from build123d import *

# Parameters (mm, degrees)
CYLINDER948_R           = 0.9
CYLINDER948_DEPTH       = 15
CYLINDER948_ROLL_ANGLE  = 90
CYLINDER949_R           = 0.9
CYLINDER949_DEPTH       = 15
CYLINDER949_ROLL_ANGLE  = 90
CYLINDER947_R           = 1.25
CYLINDER947_DEPTH       = 10
CYLINDER947_PITCH_ANGLE = 90
CYLINDER946_R           = 1.25
CYLINDER946_DEPTH       = 10
CYLINDER946_PITCH_ANGLE = 90
BOX556_W                = 8
BOX556_H                = 15
BOX556_DEPTH            = 20


with BuildPart() as cylinder1099:
    # Cylinder948 → Cylinder948 (new body)
    with BuildSketch(Plane.XY):
        Circle(CYLINDER948_R)
    extrude(amount=CYLINDER948_DEPTH)


with BuildPart() as cylinder1099_1:
    # Cylinder948 roll: moved
    add(cylinder1099.part.rotate(Axis((0, 0, 0), (1, 0, 0)), CYLINDER948_ROLL_ANGLE))


with BuildPart() as cylinder1099_2:
    # Cylinder948 placement: moved
    add(cylinder1099_1.part.moved(Location((27, 85, -10.2))))


with BuildPart() as fusion595:
    # Cylinder949 → Cylinder949 (new body)
    with BuildSketch(Plane.XY):
        Circle(CYLINDER949_R)
    extrude(amount=CYLINDER949_DEPTH)


with BuildPart() as fusion595_1:
    # Cylinder949 roll: moved
    add(fusion595.part.rotate(Axis((0, 0, 0), (1, 0, 0)), CYLINDER949_ROLL_ANGLE))


with BuildPart() as fusion595_2:
    # Cylinder949 placement: moved
    add(fusion595_1.part.moved(Location((27, 85, 0))))

    # Fusion595: union Cylinder1099
    add(cylinder1099_2.part)


with BuildPart() as fusion595_3:
    # Fusion595 placement: moved
    add(fusion595_2.part.moved(Location((-4.2, 9.5, -5.9))))


with BuildPart() as cylinder1094:
    # Cylinder947 → Cylinder947 (new body)
    with BuildSketch(Plane.XY):
        Circle(CYLINDER947_R)
    extrude(amount=CYLINDER947_DEPTH)


with BuildPart() as cylinder1094_1:
    # Cylinder947 pitch: moved
    add(cylinder1094.part.rotate(Axis((0, 0, 0), (0, 1, 0)), CYLINDER947_PITCH_ANGLE))


with BuildPart() as cylinder1094_2:
    # Cylinder947 placement: moved
    add(cylinder1094_1.part.moved(Location((13.5, 83, -11))))


with BuildPart() as fusion594:
    # Cylinder946 → Cylinder946 (new body)
    with BuildSketch(Plane.XY):
        Circle(CYLINDER946_R)
    extrude(amount=CYLINDER946_DEPTH)


with BuildPart() as fusion594_1:
    # Cylinder946 pitch: moved
    add(fusion594.part.rotate(Axis((0, 0, 0), (0, 1, 0)), CYLINDER946_PITCH_ANGLE))


with BuildPart() as fusion594_2:
    # Cylinder946 placement: moved
    add(fusion594_1.part.moved(Location((13.5, 91, -11))))

    # Fusion594: union Cylinder1094
    add(cylinder1094_2.part)


with BuildPart() as fusion594_3:
    # Fusion594 placement: moved
    add(fusion594_2.part.moved(Location((4, 0, 0))))


with BuildPart() as steering_servo_front_mount:
    # Box556 → Box556 (new body)
    with BuildSketch(Plane(origin=(19.5, 79.5, -21), x_dir=(1, 0, 0), z_dir=(0, 0, 1))):
        with Locations((4, 7.5)):
            Rectangle(BOX556_W, BOX556_H)
    extrude(amount=BOX556_DEPTH)

    # Cut693: cut Fusion594
    add(fusion594_3.part, mode=Mode.SUBTRACT)

    # Cut694: cut Fusion595
    add(fusion595_3.part, mode=Mode.SUBTRACT)


solid = steering_servo_front_mount.part
For this review, take the finished solid that the model builds, in its own axes (mm). Coordinates: 2 decimals unless noted, no trailing zeros. Order: outer loops, then holes, each group sorted by start corner. A loop starts at its lowest first (then second) coordinate and runs counter-clockwise, first axis right, second up. Notation, with made-up numbers: (19, -37.5) -> (31, -37.5) arc R11 cw to (31, -20.5) -> close; hole circle Ø1 at (15.5, 18). An arc over 180 degrees is marked (long way). Return JSON: item names as keys, results as strings.
1. We need section B-B on z = -16.1. Write out the cut boundary in (x, y), and give its area (3 significant figures).
Answer block:
{"outline": "(19.5, 79.5) -> (21.9, 79.5) -> (21.9, 94.5) -> (19.5, 94.5) -> close; (23.7, 79.5) -> (27.5, 79.5) -> (27.5, 94.5) -> (23.7, 94.5) -> close", "area": "93.0 mm²"}
2. We need section C-C on x = 22.8. Write out the cut boundary in (y, z), and give its area (3 significant figures).
Answer block:
{"outline": "(79.5, -21) -> (94.5, -21) -> (94.5, -17) -> (79.5, -17) -> close; (79.5, -15.2) -> (94.5, -15.2) -> (94.5, -6.8) -> (79.5, -6.8) -> close; (79.5, -5) -> (94.5, -5) -> (94.5, -1) -> (79.5, -1) -> close; hole circle Ø2.5 at (83, -11); hole circle Ø2.5 at (91, -11)", "area": "236 mm²"}
3. We need section A-A on y = 83. Write out the cut boundary in (x, z).
Answer block:
{"outline": "(19.5, -21) -> (27.5, -21) -> (27.5, -12.25) -> (19.5, -12.25) -> close; (19.5, -9.75) -> (27.5, -9.75) -> (27.5, -1) -> (19.5, -1) -> close; hole circle Ø1.8 at (22.8, -16.1); hole circle Ø1.8 at (22.8, -5.9)"}
4. The part is to be moulded in two halves that separate along X. For faces 1 (the flat face through (27.5, 87, -11)), 2 (the cylindrical face through (23.44, 92.24, -10.84)), 3 (the cylindrical face through (23.215, 87.105, -6.698)), say which applies: +X half, -X half, draft (parallel to the pull), parting line (faces both ways), or undercut.
Answer block:
{"face 1": "+X half", "face 2": "draft", "face 3": "undercut"}
5. For line 1 (Z direction, x = 22.8, y = 85.5); line 2 (Y direction, x = 23, z = -11); line 3 (Y direction, x = 20, z = -11.75), list the stretches that pass through material, from the lowest coordinate up. Write a range as from..to.
Answer block:
{"line 1": "-21..-17, -15.2..-6.8, -5..-1", "line 2": "79.5..81.75, 84.25..89.75, 92.25..94.5", "line 3": "79.5..82, 84..90, 92..94.5"}
6. We need section D-D on z = -11. Write out the cut boundary in (x, y).
Answer block:
{"outline": "(19.5, 79.5) -> (27.5, 79.5) -> (27.5, 81.75) -> (19.5, 81.75) -> close; (19.5, 84.25) -> (27.5, 84.25) -> (27.5, 89.75) -> (19.5, 89.75) -> close; (19.5, 92.25) -> (27.5, 92.25) -> (27.5, 94.5) -> (19.5, 94.5) -> close"}
